```python
from build123d import *

# Parameters (mm, degrees)
F0_W     = 49
F0_H     = 29
F1_DEPTH = 3
F2_R     = 1.55
F3_DEPTH = 25.4
F4_R     = 2


with BuildPart() as f1:
    # F0 (on Top) → F1 (new body)
    with BuildSketch(Plane.XY):
        Rectangle(F0_W, F0_H)
    extrude(amount=F1_DEPTH)

    # F2 (on face) → F3 (cut)
    with BuildSketch(Plane.XY.offset(3)):
        with Locations((-4.5, -8.5)):
            Circle(F2_R)
        with Locations((-4.5, 8.5)):
            Circle(F2_R)
    extrude(amount=-F3_DEPTH, mode=Mode.SUBTRACT)

    # F4
    f4_edges = [f1.edges().sort_by_distance(p)[0] for p in [
        (-24.5, 14.5, 1.5),
        (-24.5, -14.5, 1.5),
        (24.5, -14.5, 1.5),
        (24.5, 14.5, 1.5),
    ]]
    fillet(f4_edges, radius=F4_R)


solid = f1.part
```
The listing builds one solid part. Answer for the finished solid, in the listing's coordinates (mm). Round coordinates to 2 decimals unless told otherwise and drop trailing zeros. Loops run counter-clockwise (first coordinate to the right, second up) from the corner with the lowest first, then second, coordinate; pieces in that order, holes last.
Q1. Section A-A, the plane y = -8.5 is taken. Determine the outline of the cut face in (x, z).
Q2. Find the intervals of material crossed by line 1 (Y direction, x = -4.5, z = 1.8); line 2 (X direction, y = -9.5, z = 2.6); line 3 (Y direction, x = -5.5, z = 2.2), in increasing order.
Q3. Given pin 1 Ø4 at (x, y) = (-4.5, 8.5) entering from +Z, flat-ended and moving along its own axis, determine where the tip first touches the part or whether it passes through.
Q4. Section B-B, the plane x = -4.5 is taken. Determine the outline of the cut face in (y, z), then the cut area to 3 significant figures.
Q5. For a pull along X with two mould halves and no side action, classify faces 1 (the face through (0, 0, 0)), 2 (the face through (23.9, 13.93, 1.52)), 3 (the face through (-5.73, 7.56, 1.52)), 4 (the face through (-5.73, -9.44, 1.52)) as released by +X, released by -X, zero draft, split by the parting line, or undercut.
Q6. Section C-C, the plane y = 8 is taken. Determine the outline of the cut face in (x, z), then the cut area to 3 significant figures.
Completed:
1. outline: (-24.5, 0) - (-6.05, 0) - (-6.05, 3) - (-24.5, 3) - close; (-2.95, 0) - (24.5, 0) - (24.5, 3) - (-2.95, 3) - close
2. line 1: y = -14.5 to -10.05, -6.95 to 6.95, 10.05 to 14.5
2. line 2: x = -24.5 to -5.68, -3.32 to 24.5
2. line 3: y = -14.5 to -9.68, -7.32 to 7.32, 9.68 to 14.5
3. pin 1: stops at z = 3
4. outline: (-14.5, 0) - (-10.05, 0) - (-10.05, 3) - (-14.5, 3) - close; (-6.95, 0) - (6.95, 0) - (6.95, 3) - (-6.95, 3) - close; (10.05, 0) - (14.5, 0) - (14.5, 3) - (10.05, 3) - close
4. area: 68.4 mm2
5. face 1: zero draft
5. face 2: released by +X
5. face 3: undercut
5. face 4: undercut
6. outline: (-24.5, 0) - (-5.97, 0) - (-5.97, 3) - (-24.5, 3) - close; (-3.03, 0) - (24.5, 0) - (24.5, 3) - (-3.03, 3) - close
6. area: 138 mm2
